from build123d import *

# Parameters (mm, degrees)
F0_R     = 2
F0_R_2   = 16
F0_R_3   = 12
F1_DEPTH = 15
F2_T     = -1.3
F3_R     = 16
F4_DEPTH = 13.7


with BuildPart() as f1:
    # F0 (on Right) → F1 (new body)
    with BuildSketch(Plane.YZ):
        with BuildLine():
            Line((0, 27.04), (-25, 27.04))
            Line((-25, 27.04), (-25, 7.54))
            Line((-25, 7.54), (-23.5, 7.54))
            ThreePointArc((-23.5, 7.54), (-22.6893076327, 7.1254723611), (-22.5507240512, 6.2255557713))
            ThreePointArc((-22.5507240512, 6.2255557713), (-23.560917154, -4.2802307332), (-19.9204959385, -14.1867625963))
            ThreePointArc((-19.9204959385, -14.1867625963), (-19.6037904967, -15.4335268949), (-20.1118893252, -16.6152879255))
            Line((-20.1118893252, -16.6152879255), (-20.6000079963, -17.1569339704))
            ThreePointArc((-20.6000079963, -17.1569339704), (-20.3430660296, -22.1000079963), (-15.3999920037, -21.8430660296))
            Line((-15.3999920037, -21.8430660296), (-15.2488749918, -21.6753774394))
            ThreePointArc((-15.2488749918, -21.6753774394), (-14.0358697185, -21.0329527273), (-12.6944101233, -21.3237747657))
            ThreePointArc((-12.6944101233, -21.3237747657), (-6.6080004607, -24.0624425834), (0, -25))
            ThreePointArc((0, -25), (18.0346887969, -17.7360763487), (26, 0))
            ThreePointArc((26, 0), (24.8756586881, 8.6516449625), (20.9547141799, 16.4453153497))
            ThreePointArc((20.9547141799, 16.4453153497), (20.5678212068, 17.7298278052), (21.0796574448, 18.969860904))
            Line((21.0796574448, 18.969860904), (22.6000079963, 20.6569339704))
            ThreePointArc((22.6000079963, 20.6569339704), (22.3430660296, 25.6000079963), (17.3999920037, 25.3430660296))
            Line((17.3999920037, 25.3430660296), (15.9178980328, 23.6984447825))
            ThreePointArc((15.9178980328, 23.6984447825), (14.7273428061, 23.0592399542), (13.4020450466, 23.3230398953))
            ThreePointArc((13.4020450466, 23.3230398953), (6.9539665632, 26.0935467981), (0, 27.04))
        make_face()
        with Locations((-18, -19.5)):
            Circle(F0_R, mode=Mode.SUBTRACT)
        Circle(F0_R_2, mode=Mode.SUBTRACT)
        with Locations((20, 23)):
            Circle(F0_R, mode=Mode.SUBTRACT)
        Circle(F0_R_2)
        Circle(F0_R_3, mode=Mode.SUBTRACT)
        Circle(F0_R_3)
    extrude(amount=F1_DEPTH)

    # F2
    f2_openings = [f1.faces().sort_by_distance(p)[0] for p in [
        (7.5, -25, 17.29),
    ]]
    offset(amount=F2_T, openings=f2_openings)

    # F3 (on face) → F4 (cut, through all)
    with BuildSketch(Plane.YZ.offset(15)):
        Circle(F3_R)
    extrude(amount=-F4_DEPTH, mode=Mode.SUBTRACT)


solid = f1.part
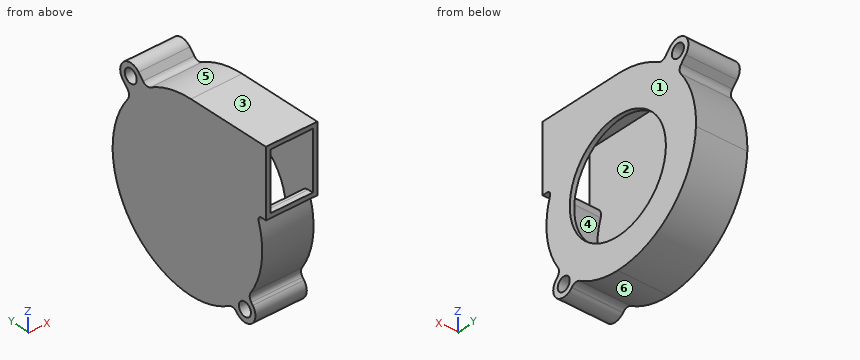
Input: part model. Units: mm. Frame: model coordinates. Face numbers are marked on the shaded views. A direction names the side the tool comes from. Give positions to 0.01 mm unless a question says otherwise; leave off trailing zeros. Order: outer loops, then holes, each group sorted by start corner. A loop starts at its lowest first (then second) coordinate and runs counter-clockwise, first axis right, second up.
Q1. Section C-C on x = 4.5. State how many separate pieces and enclosed holes the cut face has, and give its area (3 significant figures).
Checked values:
separate pieces: 1
enclosed holes: 2
area: 239 mm2
Q2. Draft query along X for the marked faces 1, 2 and 3. Return one class per face: +X half, -X half, draft (parallel to the pull), parting line (faces both ways), or undercut.
Checked values:
face 1: +X half
face 2: undercut
face 3: draft
Q3. Section B-B on y = -1.5. Output: boundary loops of the cut face in (x, z).
Checked values:
outline: (0, -24.95) - (15, -24.95) - (15, -15.93) - (13.7, -15.93) - (13.7, -23.65) - (1.3, -23.65) - (1.3, 25.74) - (13.7, 25.74) - (13.7, 15.93) - (15, 15.93) - (15, 27.04) - (0, 27.04) - close
Q4. Set-up query: the marked faces 4, 5 and 6. Return all of +Z, -Z, +X, -X, +Y, -Y with unobstructed straight access to the full face (end or side cutting, diameter ignored); none if empty.
Checked values:
face 4: none
face 5: +Z, +X, -X
face 6: -Z, +X, -X
Q5. Section A-A on z = -2. Output: boundary loops of the cut face in (x, y), and give its area (3 significant figures).
Checked values:
outline: (0, -23.74) - (15, -23.74) - (15, -15.87) - (13.7, -15.87) - (13.7, -22.44) - (1.3, -22.44) - (1.3, 24.53) - (13.7, 24.53) - (13.7, 15.87) - (15, 15.87) - (15, 25.84) - (0, 25.84) - close
area: 120 mm2
Q6. Contact query for flat-ended pins moving along their axis: pin 1 Ø2 at (x, y) = (3, 10) entering from -Z; pin 2 Ø3 at (x, y) = (12.5, 10) entering from +Z; pin 3 Ø6 at (x, z) = (9, 16.5) entering from -Y. Output: stop coordinate, or through.
Checked values:
pin 1: stops at z = -23.39
pin 2: stops at z = 25.61
pin 3: stops at y = 19.27
Q7. Ray query, probe 1 along Z at (x, y) = (10.25, -18); probe 2 along X at (y, z) = (-12, 23); probe 3 along Z at (x, y) = (6.5, -0.5). Return the intervals inside material, ascending.
Checked values:
probe 1: z = -23 to -21.5, -17.5 to -16.2, 25.74 to 27.04
probe 2: x = 0 to 1.3, 13.7 to 15
probe 3: z = -24.99 to -23.69, 25.74 to 27.04
